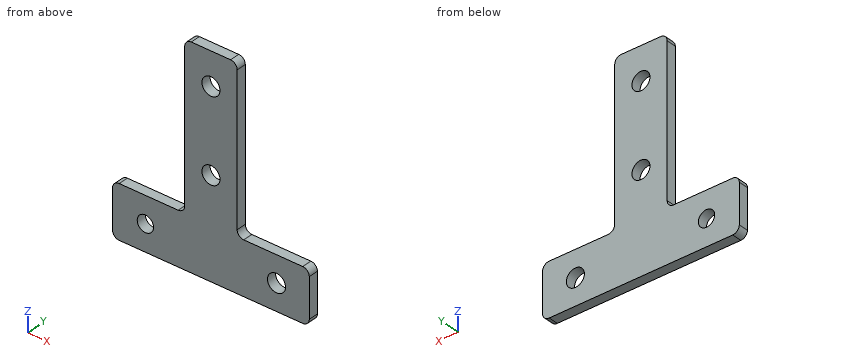
from build123d import *

# Parameters (mm, degrees)
SKETCH_1_R      = 2.485535924
SKETCH_1_R_2    = 2.75
EXTRUDE_1_DEPTH = 3


with BuildPart() as part:
    # 草图1 → 凸台-拉伸1 (new body)
    with BuildSketch(Plane(origin=(0, 0, 0), x_dir=(1, 0, 0), z_dir=(0, 1, 0))):
        with BuildLine():
            Line((0, -2), (0, -14))
            ThreePointArc((0, -14), (0.585786438, -15.414213562), (2, -16))
            Line((2, -16), (20, -16))
            ThreePointArc((20, -16), (21.414213562, -16.585786438), (22, -18))
            Line((22, -18), (22, -63))
            ThreePointArc((22, -63), (22.585786438, -64.414213562), (24, -65))
            Line((24, -65), (36, -65))
            ThreePointArc((36, -65), (37.414213562, -64.414213562), (38, -63))
            Line((38, -63), (38, -18))
            ThreePointArc((38, -18), (38.585786438, -16.585786438), (40, -16))
            Line((40, -16), (58, -16))
            ThreePointArc((58, -16), (59.414213562, -15.414213562), (60, -14))
            Line((60, -14), (60, -2))
            ThreePointArc((60, -2), (59.414213562, -0.585786438), (58, 0))
            Line((58, 0), (2, 0))
            ThreePointArc((2, 0), (0.585786438, -0.585786438), (0, -2))
        make_face()
        with Locations(Location((10, -8, 0), (0, 0, 270))):
            Circle(SKETCH_1_R, mode=Mode.SUBTRACT)
        with Locations(Location((50, -8, 0), (0, 0, 270))):
            Circle(SKETCH_1_R_2, mode=Mode.SUBTRACT)
        with Locations(Location((30, -55, 0), (0, 0, 270))):
            Circle(SKETCH_1_R_2, mode=Mode.SUBTRACT)
        with Locations(Location((30, -30, 0), (0, 0, 270))):
            Circle(SKETCH_1_R_2, mode=Mode.SUBTRACT)
    extrude(amount=EXTRUDE_1_DEPTH)


solid = part.part
Geometry: final body of the model. Coordinates: model frame, mm. Give positions to 0.01 mm unless a question says otherwise; leave off trailing zeros. Write each loop counter-clockwise with the first axis right and the second up, starting at its lowest first coordinate (ties: lowest second). Pieces come first, ordered by that corner, then holes. Notation, with made-up numbers: (-2.75, 32) - (39.25, 32) arc R19 ccw to (39.25, 42) - close; hole circle Ø6 at (13, 22). An arc over 180 degrees is marked (long way). Return JSON: item names as keys, results as strings. Group by question number.
1) Line query: line 1 (X direction, y = 2, z = 8); line 2 (X direction, y = 2.25, z = 30); line 3 (Z direction, x = 31.5, y = 2.75). Output: solid intervals per line, ascending.
2) Section D-D on y = 2.15. Return the cut outline in (x, z).
3) Section C-C on z = 30. Return the cut outline in (x, y).
4) First-contact query: P1, Ø0.9, axis at x = 13, y = 1, coming from the +Z side; P2, Ø4.5, axis at x = 30, z = 55, coming from the +Y side; P3, Ø0.9, axis at y = 1.5, z = 38.5, coming from the +X side. Flat tips, straight axial feed; report the tip coordinate or a pass-through.
5) Section A-A on x = 10. Return the cut outline in (y, z).
6) Section B-B on x = 30. Return the cut outline in (y, z), plus the area to 3 significant figures.
Filled in:
{
 "1": {"line 1": "x = 0 to 7.51, 12.49 to 47.25, 52.75 to 60", "line 2": "x = 22 to 27.25, 32.75 to 38", "line 3": "z = 0 to 27.7, 32.3 to 52.7, 57.3 to 65"},
 "2": {"outline": "(0, 2) arc R2 ccw to (2, 0) - (58, 0) arc R2 ccw to (60, 2) - (60, 14) arc R2 ccw to (58, 16) - (40, 16) arc R2 cw to (38, 18) - (38, 63) arc R2 ccw to (36, 65) - (24, 65) arc R2 ccw to (22, 63) - (22, 18) arc R2 cw to (20, 16) - (2, 16) arc R2 ccw to (0, 14) - close; hole circle Ø4.97 at (10, 8); hole circle Ø5.5 at (30, 30); hole circle Ø5.5 at (30, 55); hole circle Ø5.5 at (50, 8)"},
 "3": {"outline": "(22, 0) - (27.25, 0) - (27.25, 3) - (22, 3) - close; (32.75, 0) - (38, 0) - (38, 3) - (32.75, 3) - close"},
 "4": {"P1": "stops at z = 16", "P2": "passes through", "P3": "stops at x = 38"},
 "5": {"outline": "(0, 0) - (3, 0) - (3, 5.51) - (0, 5.51) - close; (0, 10.49) - (3, 10.49) - (3, 16) - (0, 16) - close"},
 "6": {"outline": "(0, 0) - (3, 0) - (3, 27.25) - (0, 27.25) - close; (0, 32.75) - (3, 32.75) - (3, 52.25) - (0, 52.25) - close; (0, 57.75) - (3, 57.75) - (3, 65) - (0, 65) - close", "area": "162 mm^2"}
}
